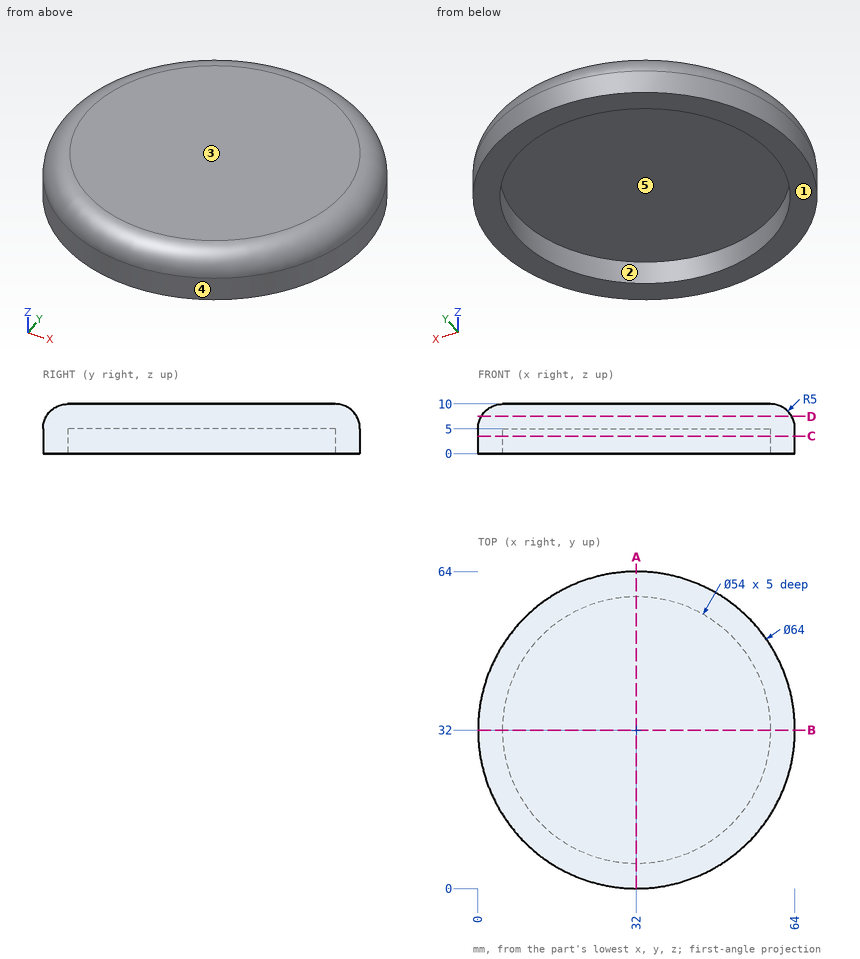
For this review, use the dimensioned drawing (mm, ordinates from the lowest corner) and the shaded views. A direction names the side the tool comes from. Round coordinates to 2 decimals unless told otherwise and drop trailing zeros. Write each loop counter-clockwise with the first axis right and the second up, starting at its lowest first coordinate (ties: lowest second). Pieces come first, ordered by that corner, then holes. Notation, with made-up numbers: M -5,80 L 11,80 A21 ccw 11,109 Z; hole C 74,39.5 d10. An arc over 180 degrees is marked long. Use CSV: the item, a comma, the result in double quotes. Start each with the question number.
(1) We need section C-C, the plane z = 3.5. State the section outline as (x, y) points.
(2) We need section A-A, the plane x = 32. State the section outline as (y, z) points, then the cut area to 3 significant figures.
(3) Tool access review of the marked faces 1 and 2: name each direction out of +Z, -Z, +X, -X, +Y, -Y from which nothing blocks a thin tool from reaching the whole face with its end or side.
(4) For line 1 along Y through (x, z) = (32, 2.8); line 2 along Z through (x, y) = (47.5, 36); line 3 along Y through (x, z) = (50, 1.25), list the stretches that pass through material, from the lowest coordinate up.
(5) We need section D-D, the plane z = 7.5. State the section outline as (x, y) points, then the cut area to 3 significant figures.
(6) Clearance check with flat-ended pins moving along their axes: P1, Ø6, axis at y = 10, z = 8, coming from the +X side; P2, Ø6, axis at x = 41.5, y = 32, coming from the -Z side; P3, Ø6, axis at y = 19.5, z = 5.5, coming from the -X side. State where each tip first meets the part, or that it passes through.
(7) The part is to be moulded in two halves that separate along Y. For the marked faces 3, 4 and 5, say which applies: +Y half, -Y half, draft (parallel to the pull), parting line (faces both ways), or undercut.
Findings:
1,outline,"C 32,32 d64; hole C 32,32 d54"
2,outline,"M 0,0 L 5,0 L 5,5 L 59,5 L 59,0 L 64,0 L 64,5 A5 ccw 59,10 L 5,10 A5 ccw 0,5 Z"
2,area,"359 mm^2"
3,face 1,"-Z, +X, -X, +Y, -Y"
3,face 2,"-Z"
4,line 1,"0 to 5, 59 to 64"
4,line 2,"5 to 10"
4,line 3,"5.54 to 11.88, 52.12 to 58.46"
5,outline,"C 32,32 d62.66"
5,area,"3,080 mm^2"
6,P1,"x = 57.16"
6,P2,"z = 5"
6,P3,"x = 1.45"
7,face 3,"draft"
7,face 4,"parting line"
7,face 5,"undercut"
